Geometry: final body of the model. Coordinates: model frame, mm. A direction names the side the tool comes from. Give positions to 0.01 mm unless a question says otherwise; leave off trailing zeros. Write each loop counter-clockwise with the first axis right and the second up, starting at its lowest first coordinate (ties: lowest second). Pieces come first, ordered by that corner, then holes.
Q1. Section A-A (y = 0). Return the cut outline in (x, z).
Q2. Mould query, pull axis Y, two halves, no side actions, for faces 3 (the cylindrical face through (23.846, 7.509, 1.479)), 4 (the flat face through (-10, 29, 12)), 5 (the cylindrical face through (-4.88, 37.18, 0.99)). Classes: +Y half, -Y half, draft (parallel to the pull), parting line (faces both ways), or undercut.
Q3. Reachability of faces 1 (the flat face through (-11.3, 22.5, 3)), 2 (the flat face through (24, -8, 0)) from +Z, -Z, +X, -X, +Y, -Y: full face, straight path, thin tool, end or side. Return the list, or none.
Q4. Line query: line 1 (Y direction, x = -1, z = 2); line 2 (X direction, y = -2, z = 6.75); line 3 (X direction, y = -17, z = 5.5). Output: solid intervals per line, ascending.
Q5. Pin query (flat end, axial travel): pin 1 Ø1 at (y, z) = (-6, 5.5) entering from +X; pin 2 Ø6 at (x, z) = (-21.5, 4) entering from -Y; pin 3 Ø1 at (x, z) = (-26, 1.5) entering from -Y. Return the tip coordinate at first contact, or that it passes through.
Q6. Section C-C (z = 5). Return the cut outline in (x, y).
from build123d import *

# Parameters (mm, degrees)
F0_R     = 37.5
F0_R_2   = 30.15
F0_R_3   = 25
F1_DEPTH = 3
F2_DEPTH = 12
F3_SIZE2 = 10
F3_SIZE  = 3
F4_R     = 3


with BuildPart() as f1:
    # F0 (on Top) → F1 (new body)
    with BuildSketch(Plane.XY):
        Circle(F0_R)
        Circle(F0_R_2, mode=Mode.SUBTRACT)
        Circle(F0_R_2)
        Circle(F0_R_3, mode=Mode.SUBTRACT)
    extrude(amount=F1_DEPTH)

    # F0 (on Top) → F2 (join)
    with BuildSketch(Plane.XY):
        Circle(F0_R)
        Circle(F0_R_2, mode=Mode.SUBTRACT)
    extrude(amount=F2_DEPTH)

    # F3
    f3_edges = [f1.edges().sort_by_distance(p)[0] for p in [
        (-37.5, 0, 12),
    ]]
    f3_side = f1.faces().sort_by_distance((-36.43934, 0, 12))[0]
    chamfer(f3_edges, length=F3_SIZE, length2=F3_SIZE2, reference=f3_side)

    # F4
    f4_edges = [f1.edges().sort_by_distance(p)[0] for p in [
        (-34.5, 0, 12),
    ]]
    fillet(f4_edges, radius=F4_R)


solid = f1.part
Computed:
1. outline: (-37.5, 0) - (-25, 0) - (-25, 3) - (-30.15, 3) - (-30.15, 12) - (-32.27, 12) arc R3 ccw to (-35.14, 9.86) - (-37.5, 2) - close; (25, 0) - (37.5, 0) - (37.5, 2) - (35.14, 9.86) arc R3 ccw to (32.27, 12) - (30.15, 12) - (30.15, 3) - (25, 3) - close
2. face 3: undercut
2. face 4: draft
2. face 5: parting line
3. face 1: +Z
3. face 2: -Z, +X, -X, +Y, -Y
4. line 1: y = -37.49 to -24.98, 24.98 to 37.49
4. line 2: x = -36.02 to -30.08, 30.08 to 36.02
4. line 3: x = -32.24 to -24.9, 24.9 to 32.24
5. pin 1: stops at x = 36.13
5. pin 2: stops at y = -32.21
5. pin 3: stops at y = -27.5
6. outline: circle Ø73.2 at (0, 0); hole circle Ø60.3 at (0, 0)
